Design review of the part built by this model. Coordinates are the model's own, in mm. Face numbers are marked on the shaded views. A direction names the side the tool comes from. Coordinates: 2 decimals unless noted, no trailing zeros. Write each loop counter-clockwise with the first axis right and the second up, starting at its lowest first coordinate (ties: lowest second). Pieces come first, ordered by that corner, then holes. Notation, with made-up numbers: (19, 68.25) - (77, 68.25) arc R29 ccw to (77, 95.25) - close; hole circle Ø7 at (50, 37.5). An arc over 180 degrees is marked (long way). Use a Markdown table: item, result.
from build123d import *

# Parameters (mm, degrees)
EXTRUDE_1_DEPTH     = 45.4
HOLE_WIZARD_1_D     = 2.8
HOLE_WIZARD_1_DEPTH = 3.5


with BuildPart() as part:
    # 草图1 → 凸台-拉伸1 (new body)
    with BuildSketch(Plane.XY):
        Polygon((-25.32278481, 7.405063291), (13.67721519, 7.405063291), (14.17721519, 6.905063291), (14.17721519, -2.694936709), (13.67721519, -3.194936709), (6.17721519, -3.194936709), (6.17721519, 1.905063291), (-17.82278481, 1.905063291), (-17.82278481, -3.194936709), (-25.32278481, -3.194936709), (-25.82278481, -2.694936709), (-25.82278481, 6.905063291), align=None)
    extrude(amount=EXTRUDE_1_DEPTH)

    # 孔1
    with Locations(Plane(origin=(4.17721519, 7.405063291, 12.7), x_dir=(0, 0, 1), z_dir=(0, 1, 0))):
        with Locations((0, 0), (20, 0), (0, -20), (20, -20)):
            Hole(HOLE_WIZARD_1_D / 2, depth=HOLE_WIZARD_1_DEPTH)


solid = part.part
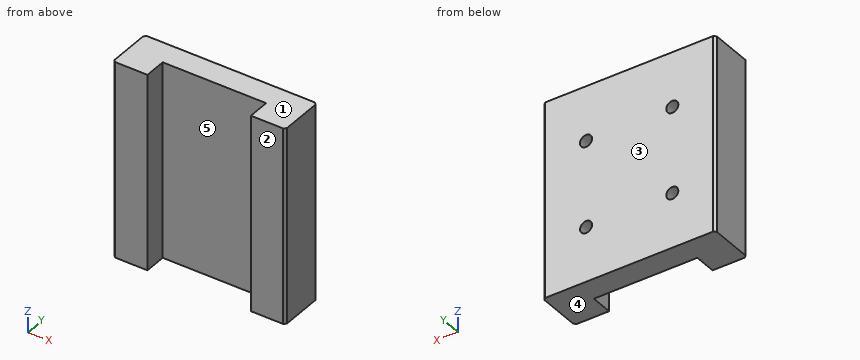
(1) Take a section at C-C on x = -11. Write out the cut boundary in (y, z), and give its area (3 significant figures).
Determined:
| item | result |
|---|---|
| outline | (1.91, 0) - (7.41, 0) - (7.41, 45.4) - (1.91, 45.4) - close |
| area | 250 mm2 |
(2) Take a section at D-D on z = 12.7. Write out the cut boundary in (x, y).
Determined:
| item | result |
|---|---|
| outline | (-25.82, -2.69) - (-25.32, -3.19) - (-17.82, -3.19) - (-17.82, 1.91) - (6.18, 1.91) - (6.18, -3.19) - (13.68, -3.19) - (14.18, -2.69) - (14.18, 6.91) - (13.68, 7.41) - (5.58, 7.41) - (5.58, 3.91) - (2.78, 3.91) - (2.78, 7.41) - (-14.42, 7.41) - (-14.42, 3.91) - (-17.22, 3.91) - (-17.22, 7.41) - (-25.32, 7.41) - (-25.82, 6.91) - close |
(3) Take a section at A-A on y = 1. Write out the cut boundary in (x, z).
Determined:
| item | result |
|---|---|
| outline | (-25.82, 0) - (-17.82, 0) - (-17.82, 45.4) - (-25.82, 45.4) - close; (6.18, 0) - (14.18, 0) - (14.18, 45.4) - (6.18, 45.4) - close |
(4) Draft analysis for pull direction Y (two halves, no side actions). For the marked faces 1, 2 and 3, state which applies: +Y half, -Y half, draft (parallel to the pull), parting line (faces both ways), or undercut.
Determined:
| item | result |
|---|---|
| face 1 | draft |
| face 2 | -Y half |
| face 3 | +Y half |
(5) For pin 1 (3.5 mm diameter, centred on x = 4.18, z = 12.7, fed in from -Y); pin 2 (1.4 mm diameter, centred on x = 4.5, z = 32.5, fed in from +Y), all flat-tipped, find the tip position at first contact; note any pin that passes through.
Determined:
| item | result |
|---|---|
| pin 1 | y = 1.91 |
| pin 2 | y = 3.91 |
(6) Take a section at B-B on z = 5. Write out the cut boundary in (x, y), and give its area (3 significant figures).
Determined:
| item | result |
|---|---|
| outline | (-25.82, -2.69) - (-25.32, -3.19) - (-17.82, -3.19) - (-17.82, 1.91) - (6.18, 1.91) - (6.18, -3.19) - (13.68, -3.19) - (14.18, -2.69) - (14.18, 6.91) - (13.68, 7.41) - (-25.32, 7.41) - (-25.82, 6.91) - close |
| area | 301 mm2 |
(7) For L1, parallel to X at y = 5.4, z = 12.7; L2, parallel to X at y = 1.5, z = 25; L3, parallel to Y at x = -12, z = 12, list the stretches that pass through material, from the lowest coordinate up. Write a range as from..to.
Determined:
| item | result |
|---|---|
| L1 | -25.82..-17.22, -14.42..2.78, 5.58..14.18 |
| L2 | -25.82..-17.82, 6.18..14.18 |
| L3 | 1.91..7.41 |
(8) Machinability: for the marked faces 4 and 5, which of the approach directions +Z, -Z, +X, -X, +Y, -Y give a long, thin tool a straight path to every point of the face, cutting with its end or side? Answer none if there is none.
Determined:
| item | result |
|---|---|
| face 4 | -Z, +X, -X, +Y, -Y |
| face 5 | +Z, -Z, -Y |
